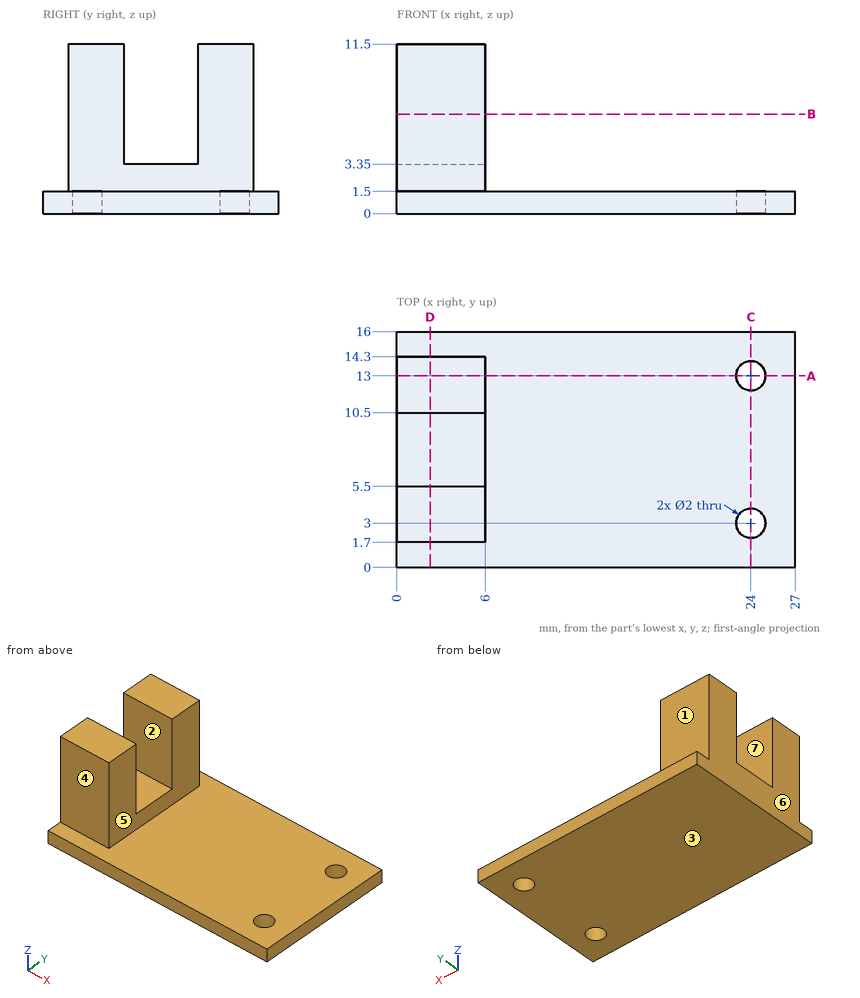
Geometry check sheet. Reference: drawing and pictorial views, mm from the part's lowest x, y, z. A direction names the side the tool comes from. Round coordinates to 2 decimals unless told otherwise and drop trailing zeros. Write each loop counter-clockwise with the first axis right and the second up, starting at its lowest first coordinate (ties: lowest second). Pieces come first, ordered by that corner, then holes.
1. Section check D-D on x = 2.25. Enter the section's corners in (y, z), plus the area to 3 significant figures.
2. Draft check along Y on the marked faces 1, 2, 3 and 4. Enter one of: +Y half, -Y half, draft (parallel to the pull), parting line (faces both ways), or undercut.
3. Section check C-C on x = 24. Enter the section's corners in (y, z).
4. Access from +Z, -Z, +X, -X, +Y, -Y to the whole of each face (thin tool, end or side, straight path). Record for the marked faces 5, 6 and 7.
5. Section check B-B on z = 6.75. Enter the section's corners in (x, y).
6. Gauge pin test, flat ends, axial feed: P1, Ø1.5, axis at x = 2.5, y = 7, coming from the +Z side; P2, Ø1.8, axis at x = 3, z = 9.5, coming from the +Y side; P3, Ø6.5, axis at x = 2, z = 6, coming from the -Y side. Record the tip position at first contact, or that the pin passes through.
7. Section check A-A on y = 13. Enter the section's corners in (x, z), plus the area to 3 significant figures.
8. Scan lines: L1, parallel to Y at x = 24, z = 0.4; L2, parallel to X at y = 13, z = 1.2; L3, parallel to Y at x = 3, z = 11. Record each from-to range of solid material in increasing order.
Answer:
1. outline: (0, 0) - (16, 0) - (16, 1.5) - (14.3, 1.5) - (14.3, 11.5) - (10.5, 11.5) - (10.5, 3.35) - (5.5, 3.35) - (5.5, 11.5) - (1.7, 11.5) - (1.7, 1.5) - (0, 1.5) - close
1. area: 109 mm2
2. face 1: +Y half
2. face 2: undercut
2. face 3: draft
2. face 4: -Y half
3. outline: (0, 0) - (2, 0) - (2, 1.5) - (0, 1.5) - close; (4, 0) - (12, 0) - (12, 1.5) - (4, 1.5) - close; (14, 0) - (16, 0) - (16, 1.5) - (14, 1.5) - close
4. face 5: +Z, +X, +Y, -Y
4. face 6: +Z, -Z, -X, +Y, -Y
4. face 7: +Z, +X, -X
5. outline: (0, 1.7) - (6, 1.7) - (6, 5.5) - (0, 5.5) - close; (0, 10.5) - (6, 10.5) - (6, 14.3) - (0, 14.3) - close
6. P1: stops at z = 3.35
6. P2: stops at y = 14.3
6. P3: stops at y = 1.7
7. outline: (0, 0) - (23, 0) - (23, 1.5) - (6, 1.5) - (6, 11.5) - (0, 11.5) - close; (25, 0) - (27, 0) - (27, 1.5) - (25, 1.5) - close
7. area: 97.5 mm2
8. L1: y = 0 to 2, 4 to 12, 14 to 16
8. L2: x = 0 to 23, 25 to 27
8. L3: y = 1.7 to 5.5, 10.5 to 14.3
